Design review of the part built by this model. Coordinates are the model's own, in mm. Face numbers are marked on the shaded views. Coordinates: 2 decimals unless noted, no trailing zeros. Write each loop counter-clockwise with the first axis right and the second up, starting at its lowest first coordinate (ties: lowest second). Pieces come first, ordered by that corner, then holes. Notation, with made-up numbers: M -36,88 L -5,88 A21 cw -5,92 Z; hole C 48,60 d5. An arc over 180 degrees is marked long. Write item = value, one per line.
```python
from build123d import *

# Parameters (mm, degrees)
SKETCH_1_R      = 19
EXTRUDE_1_DEPTH = 20
SKETCH_2_R      = 1
EXTRUDE_2_DEPTH = 90
SKETCH_3_R      = 19
EXTRUDE_3_DEPTH = 20
SKETCH_4_R      = 1
EXTRUDE_4_DEPTH = 90
SKETCH_5_R      = 19
EXTRUDE_5_DEPTH = 20


with BuildPart() as part:
    # 草图1 → 凸台-拉伸1 (new body)
    with BuildSketch(Plane.XY):
        Circle(SKETCH_1_R)
    extrude(amount=EXTRUDE_1_DEPTH)

    # 草图2 → 凸台-拉伸2 (add)
    with BuildSketch(Plane.XY.offset(20)):
        with Locations(Location((0, 0, 0), (0, 0, 180))):
            Circle(SKETCH_2_R)
    extrude(amount=EXTRUDE_2_DEPTH)

    # 草图3 → 凸台-拉伸3 (add)
    with BuildSketch(Plane.XY.offset(110)):
        Circle(SKETCH_3_R)
    extrude(amount=EXTRUDE_3_DEPTH)

    # 草图4 → 凸台-拉伸4 (add)
    with BuildSketch(Plane.XY.offset(130)):
        with Locations(Location((0, 0, 0), (0, 0, 180))):
            Circle(SKETCH_4_R)
    extrude(amount=EXTRUDE_4_DEPTH)

    # 草图5 → 凸台-拉伸5 (add)
    with BuildSketch(Plane.XY.offset(220)):
        Circle(SKETCH_5_R)
    extrude(amount=EXTRUDE_5_DEPTH)


solid = part.part
```
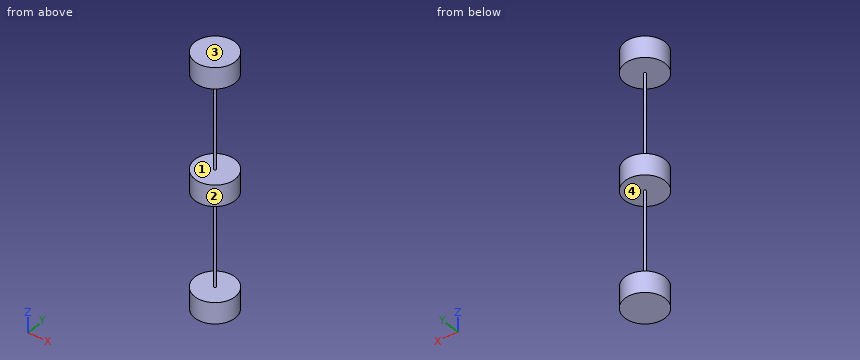
Q1. Consider section B-B, the plane x = -11.5. State the section outline as (y, z) points.
Check result:
outline = M -15.12,0 L 15.12,0 L 15.12,20 L -15.12,20 Z; M -15.12,110 L 15.12,110 L 15.12,130 L -15.12,130 Z; M -15.12,220 L 15.12,220 L 15.12,240 L -15.12,240 Z
Q2. For P1, Ø2, axis at y = 1.5, z = 58, coming from the +X side; P2, Ø1, axis at x = 2, z = 126.5, coming from the -Y side, all flat-tipped, find the tip position at first contact; note any pin that passes through.
Check result:
P1 = 0.87
P2 = -18.94
Q3. Consider section D-D, the plane z = 60. State the section outline as (x, y) points, and give its area (3 significant figures).
Check result:
outline = C 0,0 d2
area = 3.14 mm²
Q4. The part is to be moulded in two halves that separate along Z. For the marked faces 1, 2, 3 and 4, say which applies: +Z half, -Z half, draft (parallel to the pull), parting line (faces both ways), or undercut.
Check result:
face_1 = undercut
face_2 = draft
face_3 = +Z half
face_4 = undercut
Q5. Consider section A-A, the plane y = 12. State the section outline as (x, z) points, and give its area (3 significant figures).
Check result:
outline = M -14.73,0 L 14.73,0 L 14.73,20 L -14.73,20 Z; M -14.73,110 L 14.73,110 L 14.73,130 L -14.73,130 Z; M -14.73,220 L 14.73,220 L 14.73,240 L -14.73,240 Z
area = 1,770 mm²
Q6. Consider section C-C, the plane z = 127. State the section outline as (x, y) points, and give its area (3 significant figures).
Check result:
outline = C 0,0 d38
area = 1,130 mm²
Q7. Wall thickness on line 1 (Z direction, x = -3, y = 5); line 2 (X direction, y = 15.5, z = 123); line 3 (X direction, y = 7.5, z = 117): over which ranges is each line inside the solid? List them lowest first.
Check result:
line_1 = 0 to 20, 110 to 130, 220 to 240
line_2 = -10.99 to 10.99
line_3 = -17.46 to 17.46
